Part model, mm, in its own coordinate system. A direction names the side the tool comes from. Round coordinates to 2 decimals unless told otherwise and drop trailing zeros. Loops run counter-clockwise (first coordinate to the right, second up) from the corner with the lowest first, then second, coordinate; pieces in that order, holes last. Notation, with made-up numbers: (32, 78) -> (68, 78) arc R36 cw to (68, 114) -> close; hole circle Ø6 at (46.5, 69). An arc over 180 degrees is marked (long way). Use a Markdown table: item, result. Add a question column.
Item 1: Cut at A-A, the plane z = -108.6. List the corners of the cut face in (x, y), plus the area to 3 significant figures.
Item 2: Flat gauge pins, fed straight in: pin 1 (0.9 mm diameter, centred on x = 108, y = 6, fed in from -Z); pin 2 (6 mm diameter, centred on x = 81.5, z = -29, fed in from +Y); pin 3 (1.5 mm diameter, centred on x = 109, y = 6.5, fed in from +Z). Where does each tip first touch, or does it go through?
Item 3: Cut at D-D, the plane x = 108.6. State how many separate pieces and enclosed holes the cut face has, plus the area to 3 significant figures.
Item 4: Cut at B-B, the plane z = -17. List the corners of the cut face in (x, y).
Item 5: Which spindle directions (+Z, -Z, +X, -X, +Y, -Y) get a long thin tool onto all of the face, cutting with end or side? Do faces 3 (the face through (111.51, 5.67, -110.45)), 4 (the face through (9, 4, -10.001)), 5 (the face through (109, 8, -49)). Say none if no direction does.
Item 6: Cut at C-C, the plane z = -84. List the corners of the cut face in (x, y), plus the area to 3 significant figures.
Item 7: Probe line 1 (X direction, y = 5.75, z = -14); line 2 (X direction, y = 3, z = -108.6); line 3 (X direction, y = 7.5, z = -108). List the from-to ranges inside material, lowest first. Write a range as [from, to].
Item 8: Two-plate mould, pull along Z, no slides. Class faces 1 (the face through (109, 4, -12.462)), 2 (the face through (126, 2, -62)): pulls with the +Z half, pulls with the -Z half, needs draft (parallel to the pull), parting line crosses it, or undercut.
```python
from build123d import *

# Parameters (mm, degrees)
SKETCH1_W           = 126
SKETCH1_H           = 126
BOSS_EXTRUDE1_DEPTH = 5
SKETCH3_R           = 12.5
BOSS_EXTRUDE2_DEPTH = 7.5
SKETCH4_R           = 3.45
CUT_EXTRUDE1_DEPTH  = 11.5
SKETCH6_R           = 3
CUT_EXTRUDE2_DEPTH  = 179.628805068
CHAMFER1_SIZE       = 10
CHAMFER1_SIZE_2     = 7.26542528
SKETCH9_W           = 5
SKETCH9_H           = 75
BOSS_EXTRUDE4_DEPTH = 3
SKETCH10_W          = 3
SKETCH10_H          = 3
CUT_EXTRUDE4_DEPTH  = 179.370401132
SKETCH11_W          = 5
SKETCH11_H          = 108
BOSS_EXTRUDE5_DEPTH = 3
SKETCH12_W          = 3
SKETCH12_H          = 3
CUT_EXTRUDE5_DEPTH  = 179.370401132


with BuildPart() as part:
    # Sketch1 → Boss-Extrude1 (new body)
    with BuildSketch(Plane(origin=(0, 0, 0), x_dir=(1, 0, 0), z_dir=(0, 1, 0))):
        with Locations((63, 63)):
            Rectangle(SKETCH1_W, SKETCH1_H)
    extrude(amount=BOSS_EXTRUDE1_DEPTH)

    # Sketch3 → Boss-Extrude2 (add)
    with BuildSketch(Plane(origin=(0, 5, 0), x_dir=(1, 0, 0), z_dir=(0, 1, 0))):
        with Locations(Location((108.6, 108.6, 0), (0, 0, 90))):
            Circle(SKETCH3_R)
    extrude(amount=BOSS_EXTRUDE2_DEPTH)

    # Sketch4 → Cut-Extrude1 (cut)
    with BuildSketch(Plane.XZ):
        with Locations(Location((108.6, -108.6, 0), (0, 0, 270))):
            Circle(SKETCH4_R)
    extrude(amount=-CUT_EXTRUDE1_DEPTH, mode=Mode.SUBTRACT)

    # Sketch6 → Cut-Extrude2 (cut, through all)
    with BuildSketch(Plane(origin=(0, 12.5, 0), x_dir=(1, 0, 0), z_dir=(0, 1, 0))):
        with Locations(Location((108.6, 108.6, 0), (0, 0, 270))):
            Circle(SKETCH6_R)
    extrude(amount=-CUT_EXTRUDE2_DEPTH, mode=Mode.SUBTRACT)

    # Chamfer1
    # the kernel refuses this chamfer: 10, 7.26542528 mm, written as the material it takes off along each edge
    with BuildSketch(Plane(origin=(108.6, 12.5, -108.6), x_dir=(0, 0, -1), z_dir=(1, 0, 0))) as chamfer1_piece_1_section:
        Polygon((12.5, -CHAMFER1_SIZE), (12.5 - CHAMFER1_SIZE_2, 0), (12.5, 0), align=None)
    chamfer1_piece_1 = revolve(axis=Axis((108.6, 12.5, -108.6), (0, 1, 0)), mode=Mode.PRIVATE)
    chamfer1_piece_1 = split(chamfer1_piece_1, bisect_by=Plane(origin=(108.6, 5, -100.650989912), z_dir=(0, 1, 0)), keep=Keep.TOP, mode=Mode.PRIVATE)
    add(chamfer1_piece_1, mode=Mode.SUBTRACT)

    # Sketch9 → Boss-Extrude4 (add)
    with BuildSketch(Plane(origin=(0, 5, 0), x_dir=(1, 0, 0), z_dir=(0, 1, 0))):
        with Locations((108.6, 48.95817816)):
            Rectangle(SKETCH9_W, SKETCH9_H)
    extrude(amount=BOSS_EXTRUDE4_DEPTH)

    # Sketch10 → Cut-Extrude4 (cut, through all)
    with BuildSketch(Plane(origin=(0, 8, 0), x_dir=(1, 0, 0), z_dir=(0, 1, 0))):
        with Locations((108.6, 83.95817816)):
            Rectangle(SKETCH10_W, SKETCH10_H)
        with Locations((108.6, 69.958932274)):
            Rectangle(SKETCH10_W, SKETCH10_H)
        with Locations((108.6, 55.959686388)):
            Rectangle(SKETCH10_W, SKETCH10_H)
        with Locations((108.6, 41.960440502)):
            Rectangle(SKETCH10_W, SKETCH10_H)
        with Locations((108.6, 27.961194616)):
            Rectangle(SKETCH10_W, SKETCH10_H)
        with Locations((108.6, 13.96194873)):
            Rectangle(SKETCH10_W, SKETCH10_H)
    extrude(amount=-CUT_EXTRUDE4_DEPTH, mode=Mode.SUBTRACT)

    # Sketch11 → Boss-Extrude5 (add)
    with BuildSketch(Plane(origin=(0, 5, 0), x_dir=(1, 0, 0), z_dir=(0, 1, 0))):
        with Locations((8.881061813, 63)):
            Rectangle(SKETCH11_W, SKETCH11_H)
    extrude(amount=BOSS_EXTRUDE5_DEPTH)

    # Sketch12 → Cut-Extrude5 (cut, through all)
    with BuildSketch(Plane(origin=(0, 8, 0), x_dir=(1, 0, 0), z_dir=(0, 1, 0))):
        with Locations((8.881061813, 114.5)):
            Rectangle(SKETCH12_W, SKETCH12_H)
        with Locations((8.881061813, 93.900163021)):
            Rectangle(SKETCH12_W, SKETCH12_H)
        with Locations((8.881061813, 73.300326041)):
            Rectangle(SKETCH12_W, SKETCH12_H)
        with Locations((8.881061813, 52.700489062)):
            Rectangle(SKETCH12_W, SKETCH12_H)
        with Locations((8.881061813, 32.100652082)):
            Rectangle(SKETCH12_W, SKETCH12_H)
        with Locations((8.881061813, 11.500815103)):
            Rectangle(SKETCH12_W, SKETCH12_H)
    extrude(amount=-CUT_EXTRUDE5_DEPTH, mode=Mode.SUBTRACT)


solid = part.part
```
A:
| question | item | result |
|---|---|---|
| 1 | outline | (0, 0) -> (105.15, 0) -> (105.15, 11.5) -> (105.6, 11.5) -> (105.6, 12.5) -> (103.37, 12.5) -> (97.92, 5) -> (11.38, 5) -> (11.38, 8) -> (6.38, 8) -> (6.38, 5) -> (0, 5) -> close; (111.6, 11.5) -> (112.05, 11.5) -> (112.05, 0) -> (126, 0) -> (126, 5) -> (119.28, 5) -> (113.83, 12.5) -> (111.6, 12.5) -> close |
| 1 | area | 679 mm^2 |
| 2 | pin 1 | stops at z = -118.87 |
| 2 | pin 2 | stops at y = 5 |
| 2 | pin 3 | stops at z = -11.46 |
| 3 | separate pieces | 8 |
| 3 | enclosed holes | 0 |
| 3 | area | 745 mm^2 |
| 4 | outline | (0, 0) -> (126, 0) -> (126, 5) -> (111.1, 5) -> (111.1, 8) -> (106.1, 8) -> (106.1, 5) -> (11.38, 5) -> (11.38, 8) -> (6.38, 8) -> (6.38, 5) -> (0, 5) -> close |
| 5 | face 3 | -Y |
| 5 | face 4 | +Y, -Y |
| 5 | face 5 | +Z, +X, -X, +Y |
| 6 | outline | (0, 0) -> (107.1, 0) -> (107.1, 8) -> (106.1, 8) -> (106.1, 5) -> (11.38, 5) -> (11.38, 8) -> (6.38, 8) -> (6.38, 5) -> (0, 5) -> close; (110.1, 0) -> (126, 0) -> (126, 5) -> (111.1, 5) -> (111.1, 8) -> (110.1, 8) -> close |
| 6 | area | 636 mm^2 |
| 7 | line 1 | x = [6.38, 11.38], [106.1, 107.1], [110.1, 111.1] |
| 7 | line 2 | x = [0, 105.15], [112.05, 126] |
| 7 | line 3 | x = [6.38, 11.38], [99.75, 105.2], [112, 117.45] |
| 8 | face 1 | undercut |
| 8 | face 2 | needs draft |
